from build123d import *

# Parameters (mm, degrees)
SKETCH1_W                = 207
SKETCH1_H                = 106
BOSS_EXTRUDE1_DEPTH      = 35.5
SKETCH2_W                = 201
SKETCH2_H                = 100
CUT_EXTRUDE1_DEPTH       = 32
SKETCH3_W                = 204
SKETCH3_H                = 103
SKETCH3_W_2              = 201
SKETCH3_H_2              = 100
CUT_EXTRUDE2_DEPTH       = 3
M18_CLEARANCE_HOLE2_D    = 18
FILLET1_R                = 2
FILLET2_R                = 2
SKETCH6_W                = 10
SKETCH6_H                = 10
BOSS_EXTRUDE2_DEPTH      = 29
SKETCH7_W                = 10
SKETCH7_H                = 10
BOSS_EXTRUDE3_DEPTH      = 29
SKETCH8_W                = 10
SKETCH8_H                = 10
BOSS_EXTRUDE4_DEPTH      = 29
SKETCH9_W                = 10
SKETCH9_H                = 10
BOSS_EXTRUDE5_DEPTH      = 29
M3_CLEARANCE_HOLE1_D     = 3.4
M3_CLEARANCE_HOLE1_DEPTH = 26
M3_CLEARANCE_HOLE1_TIP   = 1.021463052
SKETCH12_R               = 3
CUT_EXTRUDE4_DEPTH       = 6
SKETCH13_R               = 3
CUT_EXTRUDE5_DEPTH       = 6
SKETCH14_R               = 3
CUT_EXTRUDE6_DEPTH       = 6
SKETCH15_R               = 3
CUT_EXTRUDE8_DEPTH       = 6
SKETCH17_R               = 22.5
SKETCH16_R               = 26
SKETCH18_R               = 9
CUT_EXTRUDE9_DEPTH       = 124.976812348
SKETCH19_R               = 9
CUT_EXTRUDE10_DEPTH      = 124.976812348
SKETCH20_W               = 6
SKETCH20_H               = 11
CUT_EXTRUDE13_DEPTH      = 2
SKETCH21_W               = 6
SKETCH21_H               = 11
CUT_EXTRUDE14_DEPTH      = 2
SKETCH22_W               = 218.453693545
SKETCH22_H               = 118.706912719
SKETCH22_R               = 34.681443639
CUT_EXTRUDE15_DEPTH      = 122.579192299
SKETCH23_R               = 34.681443639
CUT_EXTRUDE16_DEPTH      = 9
CUT_EXTRUDE16_DEPTH_BACK = 3.5
M3X0_5_TAPPED_HOLE1_D    = 2.5


with BuildPart() as part:
    # Sketch1 → Boss-Extrude1 (new body)
    with BuildSketch(Plane(origin=(0, 0, 0), x_dir=(1, 0, 0), z_dir=(0, 1, 0))):
        Rectangle(SKETCH1_W, SKETCH1_H)
    extrude(amount=BOSS_EXTRUDE1_DEPTH)

    # Sketch2 → Cut-Extrude1 (cut)
    with BuildSketch(Plane(origin=(0, 35.5, 0), x_dir=(1, 0, 0), z_dir=(0, 1, 0))):
        Rectangle(SKETCH2_W, SKETCH2_H)
    extrude(amount=-CUT_EXTRUDE1_DEPTH, mode=Mode.SUBTRACT)

    # Sketch3 → Cut-Extrude2 (cut)
    with BuildSketch(Plane(origin=(0, 35.5, 0), x_dir=(1, 0, 0), z_dir=(0, 1, 0))):
        Rectangle(SKETCH3_W, SKETCH3_H)
        Rectangle(SKETCH3_W_2, SKETCH3_H_2, mode=Mode.SUBTRACT)
    extrude(amount=-CUT_EXTRUDE2_DEPTH, mode=Mode.SUBTRACT)

    # M18 Clearance Hole2 (through all)
    with Locations(Plane(origin=(64.5, 3.5, 5), x_dir=(0, 0, 1), z_dir=(0, 1, 0))):
        with Locations((0, 0), (0, -24)):
            Hole(M18_CLEARANCE_HOLE2_D / 2)

    # Fillet1
    fillet1_edges = [part.edges().sort_by_distance(p)[0] for p in [
        (100.5, 18, -50),
        (100.5, 18, 50),
        (-100.5, 18, 50),
        (-100.5, 18, -50),
        (0, 0, 53),
        (-103.5, 0, 0),
        (0, 0, -53),
        (103.5, 0, 0),
        (103.5, 17.75, 53),
        (-103.5, 17.75, 53),
        (-103.5, 17.75, -53),
        (103.5, 17.75, -53),
    ]]
    fillet(fillet1_edges, radius=FILLET1_R)

    # Fillet2
    fillet2_edges = [part.edges().sort_by_distance(p)[0] for p in [
        (-102, 34, 51.5),
        (-102, 34, -51.5),
        (102, 34, -51.5),
        (102, 34, 51.5),
    ]]
    fillet(fillet2_edges, radius=FILLET2_R)

    # Sketch6 → Boss-Extrude2 (add)
    with BuildSketch(Plane(origin=(0, 3.5, 0), x_dir=(1, 0, 0), z_dir=(0, 1, 0))):
        with Locations((-43.5, 45)):
            Rectangle(SKETCH6_W, SKETCH6_H)
    extrude(amount=BOSS_EXTRUDE2_DEPTH)

    # Sketch7 → Boss-Extrude3 (add)
    with BuildSketch(Plane(origin=(0, 3.5, 0), x_dir=(1, 0, 0), z_dir=(0, 1, 0))):
        with Locations((-43.5, -45)):
            Rectangle(SKETCH7_W, SKETCH7_H)
    extrude(amount=BOSS_EXTRUDE3_DEPTH)

    # Sketch8 → Boss-Extrude4 (add)
    with BuildSketch(Plane(origin=(0, 3.5, 0), x_dir=(1, 0, 0), z_dir=(0, 1, 0))):
        with Locations((95.5, 20)):
            Rectangle(SKETCH8_W, SKETCH8_H)
    extrude(amount=BOSS_EXTRUDE4_DEPTH)

    # Sketch9 → Boss-Extrude5 (add)
    with BuildSketch(Plane(origin=(0, 3.5, 0), x_dir=(1, 0, 0), z_dir=(0, 1, 0))):
        with Locations((95.5, -20)):
            Rectangle(SKETCH9_W, SKETCH9_H)
    extrude(amount=BOSS_EXTRUDE5_DEPTH)

    # M3 Clearance Hole1
    with Locations(Plane(origin=(-43.5, 32.5, -45), x_dir=(0, 0, 1), z_dir=(0, 1, 0))):
        with Locations((0, 0), (90, 0), (65, 139), (25, 139)):
            Hole(M3_CLEARANCE_HOLE1_D / 2, depth=M3_CLEARANCE_HOLE1_DEPTH)
            with Locations((0, 0, -(M3_CLEARANCE_HOLE1_DEPTH + M3_CLEARANCE_HOLE1_TIP / 2))):  # 118° drill point
                Cone(0, M3_CLEARANCE_HOLE1_D / 2, M3_CLEARANCE_HOLE1_TIP, mode=Mode.SUBTRACT)

    # Sketch12 → Cut-Extrude4 (cut)
    with BuildSketch(Plane.XZ):
        with Locations(Location((-43.5, 45, 0), (0, 0, 270))):
            Circle(SKETCH12_R)
    extrude(amount=-CUT_EXTRUDE4_DEPTH, mode=Mode.SUBTRACT)

    # Sketch13 → Cut-Extrude5 (cut)
    with BuildSketch(Plane.XZ):
        with Locations(Location((-43.5, -45, 0), (0, 0, 270))):
            Circle(SKETCH13_R)
    extrude(amount=-CUT_EXTRUDE5_DEPTH, mode=Mode.SUBTRACT)

    # Sketch14 → Cut-Extrude6 (cut)
    with BuildSketch(Plane.XZ):
        with Locations(Location((95.5, 20, 0), (0, 0, 270))):
            Circle(SKETCH14_R)
    extrude(amount=-CUT_EXTRUDE6_DEPTH, mode=Mode.SUBTRACT)

    # Sketch15 → Cut-Extrude8 (cut)
    with BuildSketch(Plane.XZ):
        with Locations(Location((95.5, -20, 0), (0, 0, 270))):
            Circle(SKETCH15_R)
    extrude(amount=-CUT_EXTRUDE8_DEPTH, mode=Mode.SUBTRACT)

    # Sketch17 → Loft2 section 0
    with BuildSketch(Plane(origin=(0, 0, 0), x_dir=(1, 0, 0), z_dir=(0, 1, 0))):
        with Locations((52.5, -5)):
            Circle(SKETCH17_R)
    # Sketch16 → Loft2 section 1
    with BuildSketch(Plane(origin=(0, -7.5, 0), x_dir=(1, 0, 0), z_dir=(0, 1, 0))):
        with Locations((52.5, -5)):
            Circle(SKETCH16_R)
    loft()

    # Sketch18 → Cut-Extrude9 (cut, through all)
    with BuildSketch(Plane.XZ.offset(7.5)):
        with Locations(Location((40.5, 5, 0), (0, 0, 90))):
            Circle(SKETCH18_R)
    extrude(amount=-CUT_EXTRUDE9_DEPTH, mode=Mode.SUBTRACT)

    # Sketch19 → Cut-Extrude10 (cut, through all)
    with BuildSketch(Plane.XZ.offset(7.5)):
        with Locations(Location((64.5, 5, 0), (0, 0, 90))):
            Circle(SKETCH19_R)
    extrude(amount=-CUT_EXTRUDE10_DEPTH, mode=Mode.SUBTRACT)

    # Sketch20 → Cut-Extrude13 (cut)
    with BuildSketch(Plane.XZ.offset(7.5)):
        with Locations((52.5, 25.32634314)):
            Rectangle(SKETCH20_W, SKETCH20_H)
    extrude(amount=-CUT_EXTRUDE13_DEPTH, mode=Mode.SUBTRACT)


with BuildPart() as cut_extrude13_kept_piece:
    # of the separate pieces the step leaves, the one the design keeps (cut_extrude13_pieces_kept)
    add(part.part.solids().sort_by_distance((-100, 35.5, -51.5))[0])

    # Sketch21 → Cut-Extrude14 (cut)
    with BuildSketch(Plane.XZ.offset(7.5)):
        with Locations((52.5, -15.32634314)):
            Rectangle(SKETCH21_W, SKETCH21_H)
    extrude(amount=-CUT_EXTRUDE14_DEPTH, mode=Mode.SUBTRACT)


with BuildPart() as cut_extrude14_kept_piece:
    # of the separate pieces the step leaves, the one the design keeps (cut_extrude14_pieces_kept)
    add(cut_extrude13_kept_piece.part.solids().sort_by_distance((-100, 35.5, -51.5))[0])

    # Sketch22 → Cut-Extrude15 (cut, through all)
    with BuildSketch(Plane.XZ):
        with Locations((2.060883901, -1.23653034)):
            Rectangle(SKETCH22_W, SKETCH22_H)
        with Locations(Location((52.5, 5, 0), (0, 0, 270))):
            Circle(SKETCH22_R, mode=Mode.SUBTRACT)
    extrude(amount=-CUT_EXTRUDE15_DEPTH, mode=Mode.SUBTRACT)

    # Sketch23 → Cut-Extrude16 (cut, two sides)
    with BuildSketch(Plane(origin=(0, 3.5, 0), x_dir=(1, 0, 0), z_dir=(0, 1, 0))) as cut_extrude16_sk:
        with Locations((52.5, -5)):
            Circle(SKETCH23_R)
    extrude(amount=CUT_EXTRUDE16_DEPTH, mode=Mode.SUBTRACT)
    extrude(cut_extrude16_sk.sketch, amount=-CUT_EXTRUDE16_DEPTH_BACK, mode=Mode.SUBTRACT)

    # M3x0.5 Tapped Hole1 (through all)
    with Locations(Plane(origin=(52.5, -7.5, 14.82634314), x_dir=(0, 0, -1), z_dir=(0, -1, 0))):
        with Locations((0, 0), (19.65268628, 0)):
            Hole(M3X0_5_TAPPED_HOLE1_D / 2)


solid = cut_extrude14_kept_piece.part
For this review, take the finished solid that the model builds, in its own axes (mm). A direction names the side the tool comes from. Round coordinates to 2 decimals unless told otherwise and drop trailing zeros. Loops run counter-clockwise (first coordinate to the right, second up) from the corner with the lowest first, then second, coordinate; pieces in that order, holes last. Notation, with made-up numbers: (72.5, -20) - (116.5, -20) arc R27 ccw to (116.5, 17) - close; hole circle Ø2 at (-19, -25.5). An arc over 180 degrees is marked (long way). Put each result on its own line as item: value. Start each with the question number.
1. Insertion check: P1, Ø3, axis at x = 70.5, y = -6.5, coming from the -Z side; P2, Ø2, axis at x = 52.5, y = -7, coming from the +Z side; P3, Ø1.6, axis at y = -6.5, z = -15.5, coming from the -X side. Each pin has a flat end and moves straight along its axis. Give the tip position at first contact, or say it passes through.
2. Consider section C-C on z = 5. State how many separate pieces and enclosed holes the cut face has, plus the area to 4 significant figures.
3. For faces 1 (the flat face through (55.5, -7, 25)), 2 (the cylindrical face through (53.554, -3.698, 15.498)), 3 (the flat face through (52, -7, -9.826)), list the 3-axis set-ups (+Z, -Z, +X, -X, +Y, -Y) from which the entire face can be reached by the end or side of a thin tool; tool diameter is ignored.
4. Mouldability with a two-part tool opening along X and no side actions: class faces 4 (the conical face through (34.47, -0.47, 18.82)), 5 (the flat face through (52, 0, 5)), 6 (the cylindrical face through (53.74, -3.7, -4.99)) as +X half, -X half, draft (parallel to the pull), parting line (faces both ways), or undercut.
5. Consider section B-B on y = -2.25. State the section outline as (x, z) points.
6. Consider section A-A on x = 52.5. State the section outline as (y, z) points.
7. For probe 1 along Z at (x, y) = (52, -2.75); probe 2 along X at (y, z) = (-2.5, 5); probe 3 along Z at (x, y) = (52, -1), list the stretches that pass through material, from the lowest coordinate up. Write a range as [from, to].
Result sheet:
1. P1: z = -14.78
1. P2: z = 19.83
1. P3: x = 36.09
2. separate pieces: 3
2. enclosed holes: 0
2. area: 93.75 mm^2
3. face 1: +Z, -Y
3. face 2: +Y, -Y
3. face 3: -Z, -Y
4. face 4: parting line
4. face 5: draft
4. face 6: undercut
5. outline: circle Ø47.1 at (52.5, 5); hole circle Ø18 at (40.5, 5); hole circle Ø2.5 at (52.5, -4.83); hole circle Ø2.5 at (52.5, 14.83); hole circle Ø18 at (64.5, 5)
6. outline: (-7.5, -9.83) - (-5.5, -9.83) - (-5.5, -20.07) - (0, -17.5) - (0, -6.08) - (-7.5, -6.08) - close; (-7.5, -3.58) - (0, -3.58) - (0, 13.58) - (-7.5, 13.58) - close; (-7.5, 16.08) - (0, 16.08) - (0, 27.5) - (-5.5, 30.07) - (-5.5, 19.83) - (-7.5, 19.83) - close
7. probe 1: [-18.78, -5.97], [-3.68, 13.68], [15.97, 28.78]
7. probe 2: [28.83, 31.5], [49.5, 55.5], [73.5, 76.17]
7. probe 3: [-17.96, -5.97], [-3.68, 13.68], [15.97, 27.96]
